The drawing under review shows one solid part. Ordinate dimensions are in mm from its lowest x, y, z. A direction names the side the tool comes from. Round coordinates to 2 decimals unless told otherwise and drop trailing zeros. Loops run counter-clockwise (first coordinate to the right, second up) from the corner with the lowest first, then second, coordinate; pieces in that order, holes last. Notation, with made-up numbers: (49.25, 64.25) - (88.25, 64.25) arc R17 ccw to (88.25, 93.25) - close; hole circle Ø3 at (16, 46.5). An arc over 180 degrees is marked (long way). Answer as CSV lines item,"result".
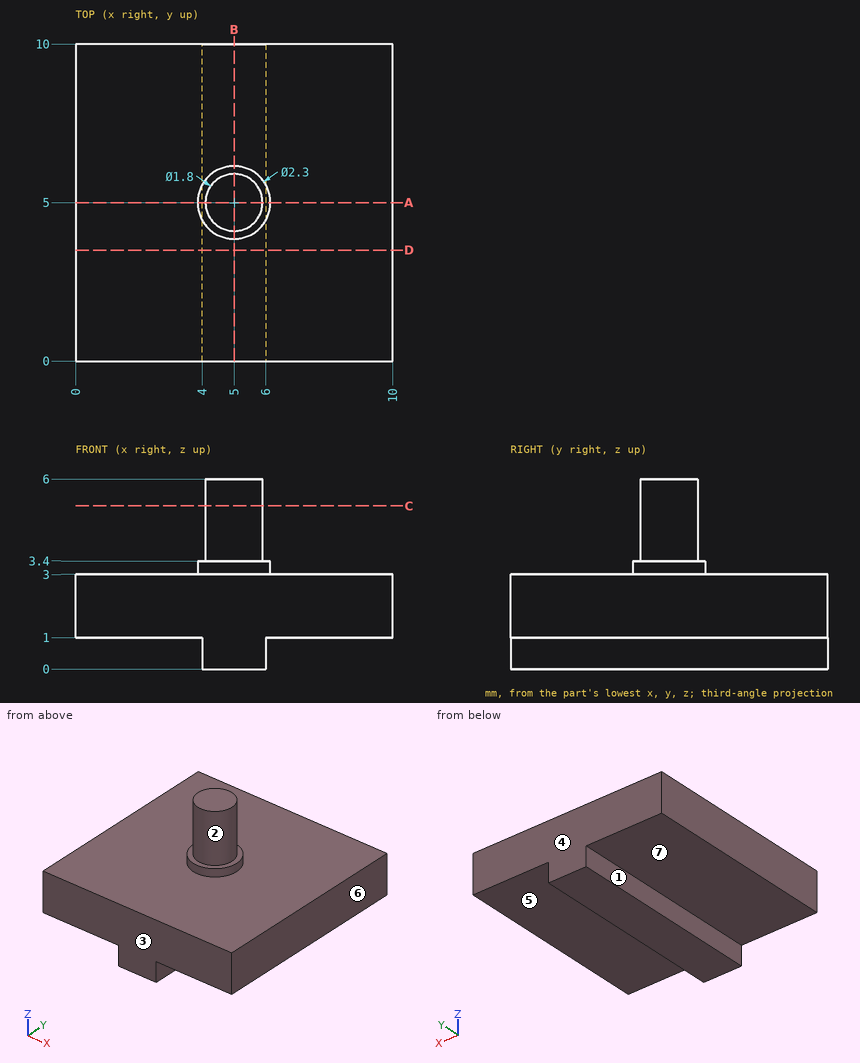
1. Take a section at D-D (y = 3.5). State the section outline as (x, z) points.
Numbers:
outline,"(0, 1) - (4, 1) - (4, 0) - (6, 0) - (6, 1) - (10, 1) - (10, 3) - (0, 3) - close"
2. Tool access review of the marked faces 5, 6 and 7: name each direction out of +Z, -Z, +X, -X, +Y, -Y from which nothing blocks a thin tool from reaching the whole face with its end or side.
Numbers:
face 5,"-Z, +X, +Y, -Y"
face 6,"+Z, -Z, +X, +Y, -Y"
face 7,"-Z, -X, +Y, -Y"
3. Draft analysis for pull direction Y (two halves, no side actions). For the marked faces 1, 2, 3 and 4, state which applies: +Y half, -Y half, draft (parallel to the pull), parting line (faces both ways), or undercut.
Numbers:
face 1,"draft"
face 2,"parting line"
face 3,"-Y half"
face 4,"+Y half"
4. Wall thickness on probe 1 along Z at (x, y) = (5.75, 7); probe 2 along X at (y, z) = (6.5, 0.8); probe 3 along Z at (x, y) = (0.5, 2.75): over which ranges is each line inside the solid? List them lowest first.
Numbers:
probe 1,"z = 0 to 3"
probe 2,"x = 4 to 6"
probe 3,"z = 1 to 3"
5. Take a section at A-A (y = 5). State the section outline as (x, z) points.
Numbers:
outline,"(0, 1) - (4, 1) - (4, 0) - (6, 0) - (6, 1) - (10, 1) - (10, 3) - (6.15, 3) - (6.15, 3.4) - (5.9, 3.4) - (5.9, 6) - (4.1, 6) - (4.1, 3.4) - (3.85, 3.4) - (3.85, 3) - (0, 3) - close"
6. Take a section at B-B (x = 5). State the section outline as (y, z) points.
Numbers:
outline,"(0, 0) - (10, 0) - (10, 3) - (6.15, 3) - (6.15, 3.4) - (5.9, 3.4) - (5.9, 6) - (4.1, 6) - (4.1, 3.4) - (3.85, 3.4) - (3.85, 3) - (0, 3) - close"
7. Take a section at C-C (z = 5.15). State the section outline as (x, y) points, plus the area to 3 significant figures.
Numbers:
outline,"circle Ø1.8 at (5, 5)"
area,"2.54 mm²"
8. Clearance check with flat-ended pins moving along their axes: pin 1 (1 mm diameter, centred on y = 6.5, z = 4.5, fed in from -X); pin 2 (2 mm diameter, centred on x = 7.5, y = 3, fed in from -Z); pin 3 (0.8 mm diameter, centred on y = 7.5, z = 0.5, fed in from -X). State where each tip first meets the part, or that it passes through.
Numbers:
pin 1,"passes through"
pin 2,"stops at z = 1"
pin 3,"stops at x = 4"
